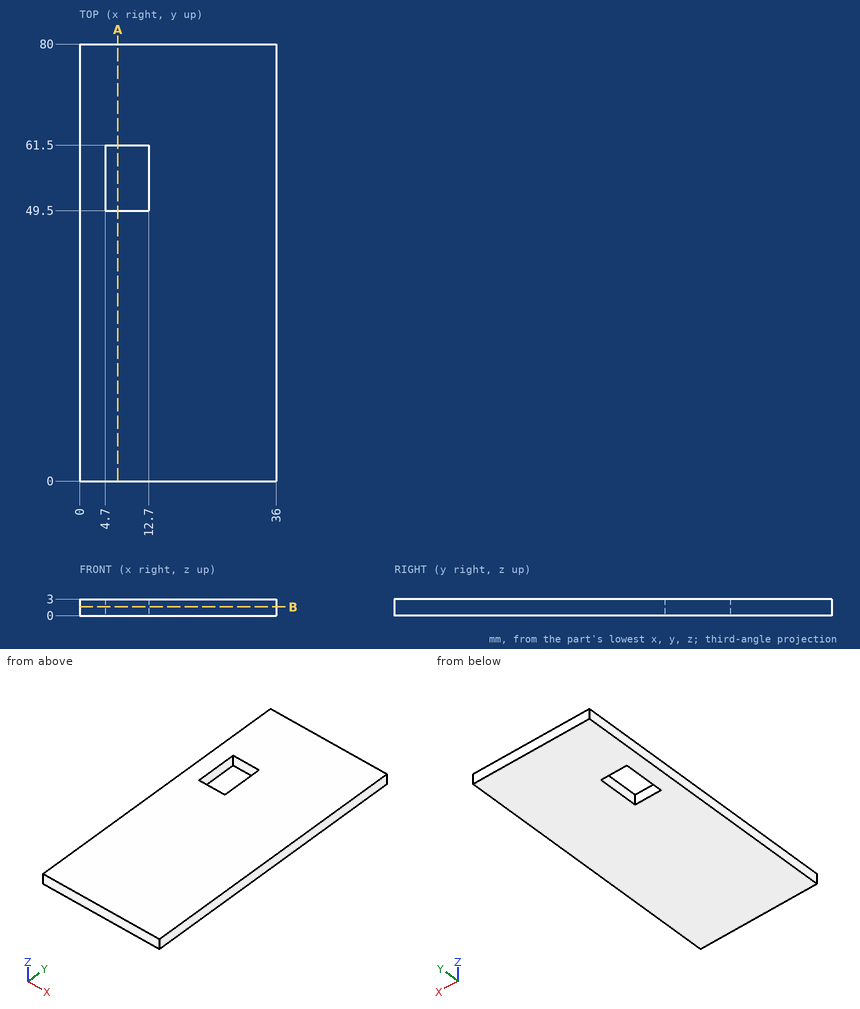
Can you work these out from the drawing? Everything is in mm from the part's minimum corner. Round coordinates to 2 decimals unless told otherwise and drop trailing zeros. Order: outer loops, then holes, each group sorted by start corner. A loop starts at its lowest first (then second) coordinate and runs counter-clockwise, first axis right, second up.
(1) If I drill on L1, parallel to X at y = 60, z = 1.45; L2, parallel to Y at x = 9, z = 1.9, over which ranges is the centre line in solid material (lowest first)?
Results are:
L1: x = 0 to 4.7, 12.7 to 36
L2: y = 0 to 49.5, 61.5 to 80
(2) I'm going to push a flat-ended pin straight in: pin 1 (1 mm diameter, centred on x = 17.5, z = 2, fed in from -Y). Where does the tip first touch, or does it pass through?
Results are:
pin 1: stops at y = 0
(3) If we section it at B-B (z = 1.6): Please give me the cut outline in (x, y), plus the area to 3 significant figures.
Results are:
outline: (0, 0) - (36, 0) - (36, 80) - (0, 80) - close; hole (4.7, 49.5) - (12.7, 49.5) - (12.7, 61.5) - (4.7, 61.5) - close
area: 2,780 mm2
(4) If we section it at A-A (x = 7): Please give me the cut outline in (y, z), plus the area to 3 significant figures.
Results are:
outline: (0, 0) - (49.5, 0) - (49.5, 3) - (0, 3) - close; (61.5, 0) - (80, 0) - (80, 3) - (61.5, 3) - close
area: 204 mm2
